from build123d import *

# Parameters (mm, degrees)
F0_W      = 14
F0_H      = 11
F1_DEPTH  = 0.5
F3_START  = -0.6
F2_W      = 1.5
F2_H      = 4
F2_W_2    = 2
F2_W_3    = 5
F3_DEPTH  = 2.4
F5_START  = -0.2
F5_DEPTH  = 0.4
F6_DEPTH  = 8
F7_R      = 0.5
F8_R      = 1
F9_R      = 0.5
F10_R     = 2
F11_R     = 0.25
F12_START = 0.5
F12_DEPTH = 3.5
F14_DEPTH = 8.5


# Not quite as in the source:
# - a feature names something its author has since deleted; it is built from what else it names


with BuildPart() as f1:
    # F0 (on Front) → F1 (new body, symmetric)
    with BuildSketch(Plane.XZ):
        Polygon((-21.05, -8.5), (21.05, -8.5), (23.95, 8.5), (-21.05, 8.5), align=None)
        with Locations((7.95, 0)):
            Rectangle(F0_W, F0_H, mode=Mode.SUBTRACT)
        with Locations((7.95, 0)):
            Rectangle(F0_W, F0_H)
    extrude(amount=F1_DEPTH, both=True)

    # F2 (on face) → F3 (join)
    with BuildSketch(Plane(origin=(0, 0.5, 0), x_dir=(-1, 0, 0), z_dir=(0, 1, 0)).offset(F3_START)):
        with Locations((25.3, 0)):
            Rectangle(F2_W, F2_H)
        with Locations((22.05, 0)):
            Rectangle(F2_W_2, F2_H)
        with Locations((23.8, 0)):
            Rectangle(F2_W, F2_H)
        with Locations((18.55, 0)):
            Rectangle(F2_W_3, F2_H)
    extrude(amount=-F3_DEPTH)

    # F2 (on face) → F5 (join)
    with BuildSketch(Plane(origin=(0, 0.5, 0), x_dir=(-1, 0, 0), z_dir=(0, 1, 0)).offset(F5_START)):
        with Locations((25.3, 0)):
            Rectangle(F2_W, F2_H)
        with Locations((22.05, 0)):
            Rectangle(F2_W_2, F2_H)
    extrude(amount=-F5_DEPTH)

    # F4 (on Top) → F6 (join, symmetric)
    with BuildSketch(Plane.XY):
        Polygon((3.95, -4), (8.95, -4), (8.95, -0.5), (6.95, -0.5), (6.95, -2), (3.95, -2), align=None)
    extrude(amount=F6_DEPTH, both=True)

    # F7
    f7_edges = [f1.edges().sort_by_distance(p)[0] for p in [
        (-21.05, 0, 8.5),
        (-21.05, 0, -8.5),
        (23.95, 0, 8.5),
        (21.05, 0, -8.5),
    ]]
    fillet(f7_edges, radius=F7_R)

    # F8
    f8_edges = [f1.edges().sort_by_distance(p)[0] for p in [
        (8.95, -4, 0),
    ]]
    fillet(f8_edges, radius=F8_R)

    # F9
    f9_edges = [f1.edges().sort_by_distance(p)[0] for p in [
        (3.95, -2, 0),
    ]]
    fillet(f9_edges, radius=F9_R)

    # F10
    f10_edges = [f1.edges().sort_by_distance(p)[0] for p in [
        (-26.05, -2.5, 0),
    ]]
    fillet(f10_edges, radius=F10_R)

    # F11
    f11_edges = [f1.edges().sort_by_distance(p)[0] for p in [
        (-24.55, 0.3, 0),
        (-23.05, 0.3, 0),
    ]]
    fillet(f11_edges, radius=F11_R)

    # F0 (on Front) → F12 (cut)
    with BuildSketch(Plane.XZ.offset(F12_START)):
        with Locations((7.95, 0)):
            Rectangle(F0_W, F0_H)
    extrude(amount=F12_DEPTH, mode=Mode.SUBTRACT)

    # F13 (on Top) → F14 (join, symmetric)
    with BuildSketch(Plane.XY):
        Polygon((-4.276, 0), (-20.55, 0), (-20.55, -2.5), align=None)
    extrude(amount=F14_DEPTH, both=True)


solid = f1.part
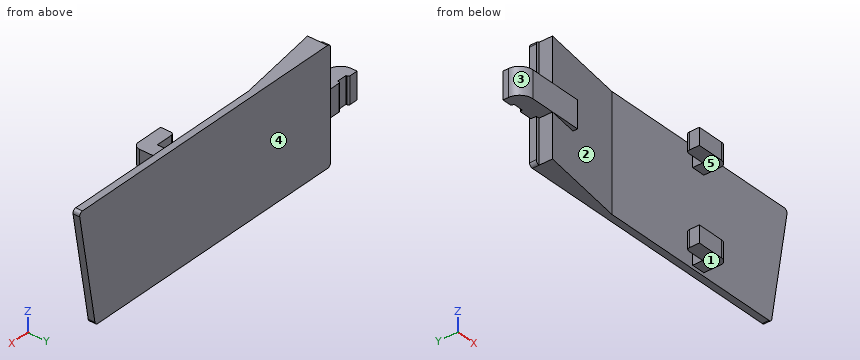
Here's how the part is built. I have some questions about the finished solid (model axes, mm). Face numbers are marked on the shaded views. A direction names the side the tool comes from. Coordinates: 2 decimals unless noted, no trailing zeros. Loops run counter-clockwise (first coordinate to the right, second up) from the corner with the lowest first, then second, coordinate; pieces in that order, holes last. Notation, with made-up numbers: (80, -18.5) -> (133, -18.5) arc R27 cw to (133, 1.5) -> close; hole circle Ø3 at (19, -6.75). An arc over 180 degrees is marked (long way). Use one line per item in the form item = value. Start each with the question number.
(1) If we section it at C-C (z = -3.25): Please give me the cut outline in (x, y).
(2) We'd pull the mould along X, two halves only. Please class the marked faces 1, 2 and 3: pulls with the +X half, pulls with the -X half, needs draft (parallel to the pull), parting line crosses it, or undercut.
(3) Please list where these lines run through material, in increasing order: line 1 along Y through (x, z) = (6, 1.5); line 2 along Y through (x, z) = (-21, 0.75); line 3 along Z through (x, y) = (-21, -2.25).
(4) On a 3-axis mill with a long thin cutter (end or side, diameter ignored), from which of +Z, -Z, +X, -X, +Y, -Y can I reach the whole of each face in a straight line? I mean the marked faces 4 and 5. Say none if no direction works.
(5) If we section it at A-A (z = 0): Please give me the cut outline in (x, y).
(6) If we section it at D-D (x = -18): Please give me the cut outline in (y, z).
(7) Will these pins go through, and if not, where does the flat tip stop? pin 1 (4.5 mm diameter, centred on x = -18.5, z = 0.5, fed in from -Y); pin 2 (6 mm diameter, centred on x = 14.5, z = -0.5, fed in from -Y); pin 3 (0.8 mm diameter, centred on x = -22.5, y = -1, fed in from -Z).
(8) If we section it at B-B (x = 14): Please give me the cut outline in (y, z).
Verdict:
q1.outline = (-21.05, -0.5) -> (-20.55, -0.5) -> (-20.55, -2.5) -> (-7.53, -0.5) -> (21.95, -0.5) -> (21.95, 0.5) -> (-21.05, 0.5) -> close
q2.face_1 = needs draft
q2.face_2 = undercut
q2.face_3 = pulls with the -X half
q3.line_1 = -0.5 to 0.5
q3.line_2 = -2.5 to 0.5
q3.line_3 = -2 to 2
q4.face_4 = +Z, -Z, +X, -X, +Y
q4.face_5 = +X, -Y
q5.outline = (-26.05, -0.5) arc R2 ccw to (-24.05, -2.5) -> (-16.05, -2.5) -> (-16.05, -1.81) -> (-7.53, -0.5) -> (22.5, -0.5) -> (22.5, 0.5) -> (-21.05, 0.5) -> (-21.05, 0.3) -> (-22.8, 0.3) arc R0.25 ccw to (-23.05, 0.05) -> (-23.05, -0.1) -> (-24.55, -0.1) -> (-24.55, 0.05) arc R0.25 ccw to (-24.8, 0.3) -> (-26.05, 0.3) -> close
q6.outline = (-2.5, -2) -> (-2.11, -2) -> (-2.11, -8.5) -> (0.5, -8.5) -> (0.5, 8.5) -> (-2.11, 8.5) -> (-2.11, 2) -> (-2.5, 2) -> close
q7.pin_1 = -2.5
q7.pin_2 = -0.5
q7.pin_3 = -2
q8.outline = (-0.5, -8.5) -> (0.5, -8.5) -> (0.5, 8.5) -> (-0.5, 8.5) -> close
